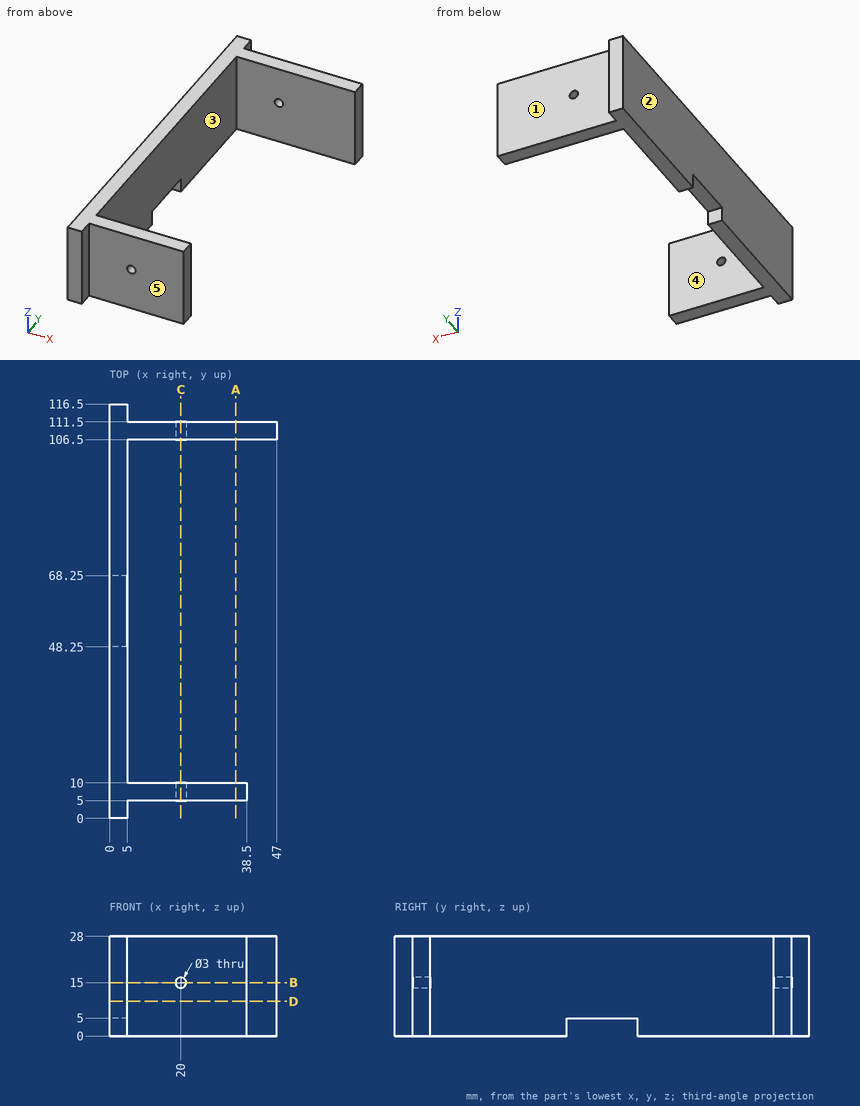
Here's the drawing with two shaded views (mm, measured from the low corner). I have some questions. A direction names the side the tool comes from. Coordinates: 2 decimals unless noted, no trailing zeros. Write each loop counter-clockwise with the first axis right and the second up, starting at its lowest first coordinate (ties: lowest second). Pieces come first, ordered by that corner, then holes. Notation, with made-up numbers: (-20, 67.5) -> (32, 67.5) arc R21 ccw to (32, 91.5) -> close; hole circle Ø2 at (45, 59). An arc over 180 degrees is marked (long way). Use a Markdown table: item, result. Add a question column.
(1) For the marked faces 4 and 5, which set-ups out of +Z, -Z, +X, -X, +Y, -Y let a thin tool reach every point of the face, with its end or its side?
(2) We'd pull the mould along Y, two halves only. Please class the marked faces 1, 2 and 3: +Y half, -Y half, draft (parallel to the pull), parting line (faces both ways), or undercut.
(3) If we section it at D-D, the plane z = 9.75: Write out the boundary of the cut face in (x, y), and give its area (3 significant figures).
(4) If we section it at B-B, the plane z = 15: Write out the boundary of the cut face in (x, y), and give its area (3 significant figures).
(5) If we section it at C-C, the plane x = 20: Write out the boundary of the cut face in (y, z), and give its area (3 significant figures).
(6) Please list where these lines run through material, in increasing order: line 1 (X direction, y = 109.6, z = 15); line 2 (X direction, y = 8.2, z = 15); line 3 (Y direction, x = 37.5, z = 18.75).
(7) If we section it at A-A, the plane x = 35.5: Write out the boundary of the cut face in (y, z), and give its area (3 significant figures).
(8) I'm going to push flat-ended pins straight in: P1, Ø1, axis at y = 40, z = 18.5, coming from the +X side; P2, Ø12, axis at y = 12.5, z = 5.5, coming from the +X side; P3, Ø14, axis at x = 25.5, z = 18.5, coming from the -Y side. Where does each tip first touch, or does it pass through?
Outcome:
| question | item | result |
|---|---|---|
| 1 | face 4 | +Z, -Z, +X |
| 1 | face 5 | +Z, -Z, +X, -Y |
| 2 | face 1 | +Y half |
| 2 | face 2 | draft |
| 2 | face 3 | undercut |
| 3 | outline | (0, 0) -> (5, 0) -> (5, 5) -> (38.5, 5) -> (38.5, 10) -> (5, 10) -> (5, 106.5) -> (47, 106.5) -> (47, 111.5) -> (5, 111.5) -> (5, 116.5) -> (0, 116.5) -> close |
| 3 | area | 960 mm^2 |
| 4 | outline | (0, 0) -> (5, 0) -> (5, 5) -> (18.5, 5) -> (18.5, 10) -> (5, 10) -> (5, 106.5) -> (18.5, 106.5) -> (18.5, 111.5) -> (5, 111.5) -> (5, 116.5) -> (0, 116.5) -> close; (21.5, 5) -> (38.5, 5) -> (38.5, 10) -> (21.5, 10) -> close; (21.5, 106.5) -> (47, 106.5) -> (47, 111.5) -> (21.5, 111.5) -> close |
| 4 | area | 930 mm^2 |
| 5 | outline | (5, 0) -> (10, 0) -> (10, 13.5) -> (5, 13.5) -> close; (5, 16.5) -> (10, 16.5) -> (10, 28) -> (5, 28) -> close; (106.5, 0) -> (111.5, 0) -> (111.5, 13.5) -> (106.5, 13.5) -> close; (106.5, 16.5) -> (111.5, 16.5) -> (111.5, 28) -> (106.5, 28) -> close |
| 5 | area | 250 mm^2 |
| 6 | line 1 | x = 0 to 18.5, 21.5 to 47 |
| 6 | line 2 | x = 0 to 18.5, 21.5 to 38.5 |
| 6 | line 3 | y = 5 to 10, 106.5 to 111.5 |
| 7 | outline | (5, 0) -> (10, 0) -> (10, 28) -> (5, 28) -> close; (106.5, 0) -> (111.5, 0) -> (111.5, 28) -> (106.5, 28) -> close |
| 7 | area | 280 mm^2 |
| 8 | P1 | stops at x = 5 |
| 8 | P2 | stops at x = 38.5 |
| 8 | P3 | stops at y = 5 |
